from build123d import *

# Parameters (mm, degrees)
CUT_EXTRUDE_2_DEPTH      = 30
CUT_EXTRUDE_2_DEPTH_BACK = 214.600093633
SKETCH_3_R               = 10


with BuildPart() as part:
    # Sketch 1 → Revolve 3 (revolve)
    with BuildSketch(Plane.XY, mode=Mode.PRIVATE) as revolve_3_sk:
        with BuildLine():
            Line((-120, 0), (-120, 25))
            Line((-120, 25), (-100, 25))
            ThreePointArc((-100, 25), (-64.644660941, 39.644660941), (-50, 75))
            Line((-50, 75), (-35, 75))
            Line((-35, 75), (-35, 25))
            Line((-35, 25), (0, 25))
            Line((0, 25), (0, 0))
            Line((0, 0), (-120, 0))
        make_face()
    revolve(revolve_3_sk.sketch.rotate(Axis((0, 0, 0), (0, 1, 0)), 270), axis=Axis((0, 0, 0), (0, 1, 0)))

    # Sketch 3 → Cut-Extrude 2 (cut, two sides: drawn at the far end of the back side and taken through both)
    with BuildSketch(Plane.XY.offset(-40).offset(-CUT_EXTRUDE_2_DEPTH_BACK)):
        with Locations(Location((0, 50, 0), (0, 0, 90))):
            Circle(SKETCH_3_R)
    extrude(amount=CUT_EXTRUDE_2_DEPTH + CUT_EXTRUDE_2_DEPTH_BACK, mode=Mode.SUBTRACT)


solid = part.part
Part model, mm, in its own coordinate system. A direction names the side the tool comes from. Give positions to 0.01 mm unless a question says otherwise; leave off trailing zeros. Write each loop counter-clockwise with the first axis right and the second up, starting at its lowest first coordinate (ties: lowest second). Pieces come first, ordered by that corner, then holes.
1) Pin check, flat tips, straight feed: pin 1 (5 mm diameter, centred on x = 48, z = -63.5, fed in from +Y); pin 2 (3 mm diameter, centred on x = 43.5, y = 39.5, fed in from -Z); pin 3 (12 mm diameter, centred on x = 0, y = 50, fed in from +Z). Stop position of each tip, or through.
Resolved:
pin 1: stops at y = 30.55
pin 2: stops at z = -50.48
pin 3: stops at z = 60.77
2) Probe L1, parallel to Z at x = 14.5, y = 41; L2, parallel to Z at x = -7, y = 32; L3, parallel to X at y = 50, z = -41. List the from-to ranges inside material, lowest first.
Resolved:
L1: z = -61.66 to -31.86, 31.86 to 61.66
L2: z = -74.16 to -34.29, 34.29 to 74.16
L3: x = -39.16 to -10, 10 to 39.16
3) Which spindle directions (+Z, -Z, +X, -X, +Y, -Y) get a long thin tool onto all of the face, cutting with end or side? Do faces 1 (the face through (10, 75, 34)), 2 (the face through (21, 50, 28)). Say none if no direction does.
Resolved:
face 1: +Z, -Z, +X, -X, +Y
face 2: +Y
4) Cut at D-D on x = -103. Write the cut outline in (y, z).
Resolved:
outline: (0, -61.57) - (25, -61.57) - (25, 61.57) - (0, 61.57) - close
5) Cut at C-C on y = 50. Write the cut outline in (x, z).
Resolved:
outline: (-10, -55.81) - (-10, -33.54) arc R35 cw (long way) to (10, -33.54) - (10, -55.81) arc R56.7 ccw (long way) to start
6) Cut at A-A on x = 0. Write the cut outline in (y, z), then the cut area to 3 significant figures.
Resolved:
outline: (0, -120) - (25, -120) - (25, -100) arc R50 cw to (40, -64.29) - (40, -35) - (25, -35) - (25, 35) - (75, 35) - (75, 50) arc R50 cw to (25, 100) - (25, 120) - (0, 120) - close; (60, -52.3) arc R50 cw to (75, -50) - (75, -35) - (60, -35) - close
area: 8,130 mm2
7) Cut at B-B on z = 0. Write the cut outline in (x, y).
Resolved:
outline: (-120, 0) - (120, 0) - (120, 25) - (100, 25) arc R50 cw to (50, 75) - (35, 75) - (35, 25) - (-35, 25) - (-35, 75) - (-50, 75) arc R50 cw to (-100, 25) - (-120, 25) - close
8) Two-plate mould, pull along X, no slides. Class faces 3 (the face through (-98, 25, 27)), 4 (the face through (-5.276, 12.675, 119.884)), 5 (the face through (0, 40, -46)): released by +X, released by -X, zero draft, split by the parting line, or undercut.
Resolved:
face 3: zero draft
face 4: split by the parting line
face 5: undercut
